The drawing under review shows one solid part. Ordinate dimensions are in mm from its lowest x, y, z. A direction names the side the tool comes from. Coordinates: 2 decimals unless noted, no trailing zeros. Write each loop counter-clockwise with the first axis right and the second up, starting at its lowest first coordinate (ties: lowest second). Pieces come first, ordered by that corner, then holes. Notation, with made-up numbers: M 2.25,75.5 L 60.25,75.5 A25 cw 60.25,88.5 Z; hole C -7.75,-5 d11. An arc over 180 degrees is marked long. Answer as CSV lines item,"result". Start each with the question number.
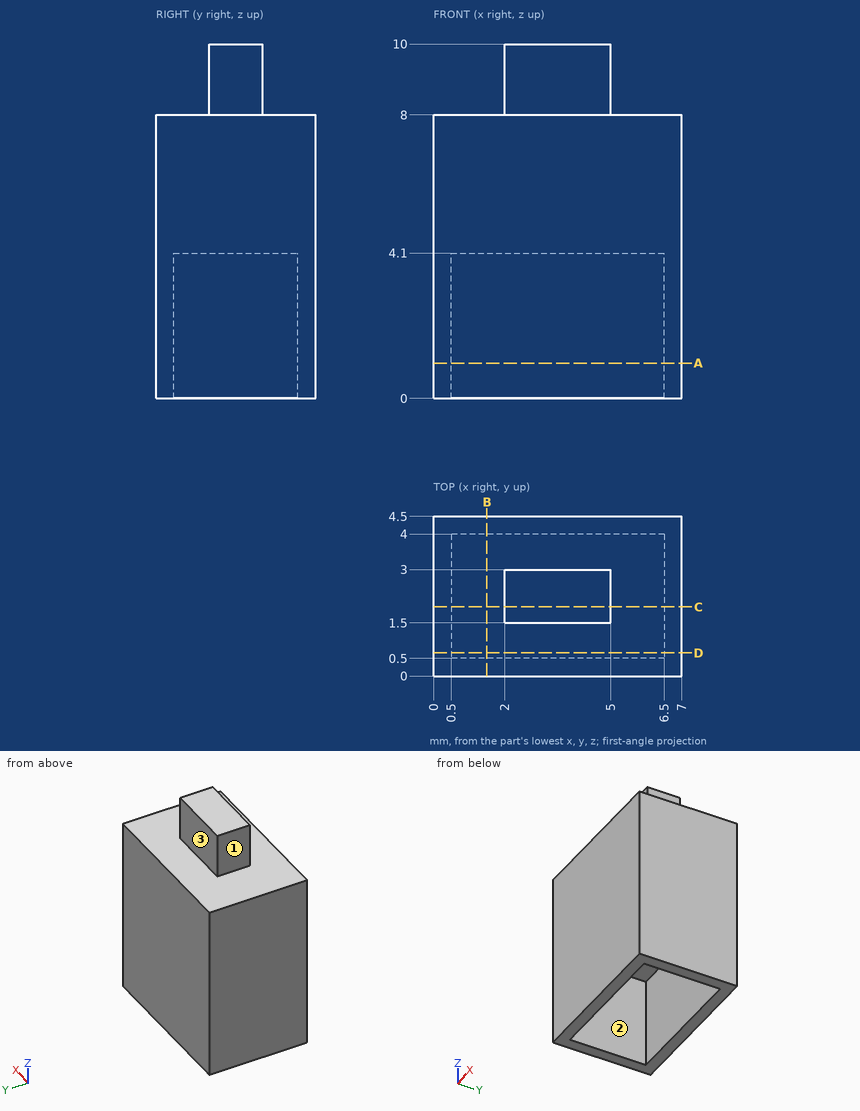
1) Clearance check with flat-ended pins moving along their axes: pin 1 Ø1.8 at (x, y) = (3.5, 2.5) entering from -Z; pin 2 Ø2 at (x, y) = (0.5, 1.5) entering from -Z; pin 3 Ø1.2 at (y, z) = (2.5, 9) entering from -X; pin 4 Ø0.6 at (x, z) = (3.5, 8.5) entering from -Y. State where each tip first meets the part, or that it passes through.
2) Take a section at D-D on y = 0.65. Give the boundary of the cut face in (x, z), and give its area (3 significant figures).
3) Tool access review of the marked faces 1, 2 and 3: name each direction out of +Z, -Z, +X, -X, +Y, -Y from which nothing blocks a thin tool from reaching the whole face with its end or side.
4) To check wall thickness, follow line 1 (X direction, y = 1.2, z = 1); line 2 (Y direction, x = 4.75, z = 3.25); line 3 (Z direction, x = 1.5, y = 2.1). State the ranges of each line that lie inside material, in increasing order. Write a range as [from, to].
5) Take a section at B-B on x = 1.5. Give the boundary of the cut face in (y, z), and give its area (4 significant figures).
6) Take a section at C-C on y = 1.95. Give the boundary of the cut face in (x, z).
7) Take a section at A-A on z = 1. Give the boundary of the cut face in (x, y), and give its area (3 significant figures).
Results:
1,pin 1,"stops at z = 4.1"
1,pin 2,"stops at z = 0"
1,pin 3,"stops at x = 2"
1,pin 4,"stops at y = 1.5"
2,outline,"M 0,0 L 0.5,0 L 0.5,4.1 L 6.5,4.1 L 6.5,0 L 7,0 L 7,8 L 0,8 Z"
2,area,"31.4 mm²"
3,face 1,"+Z, -X, +Y, -Y"
3,face 2,"-Z"
3,face 3,"+Z, +X, -X, +Y"
4,line 1,"x = [0, 0.5], [6.5, 7]"
4,line 2,"y = [0, 0.5], [4, 4.5]"
4,line 3,"z = [4.1, 8]"
5,outline,"M 0,0 L 0.5,0 L 0.5,4.1 L 4,4.1 L 4,0 L 4.5,0 L 4.5,8 L 0,8 Z"
5,area,"21.65 mm²"
6,outline,"M 0,0 L 0.5,0 L 0.5,4.1 L 6.5,4.1 L 6.5,0 L 7,0 L 7,8 L 5,8 L 5,10 L 2,10 L 2,8 L 0,8 Z"
7,outline,"M 0,0 L 7,0 L 7,4.5 L 0,4.5 Z; hole M 0.5,0.5 L 6.5,0.5 L 6.5,4 L 0.5,4 Z"
7,area,"10.5 mm²"
